from build123d import *

# Parameters (mm, degrees)
F1_DEPTH = 12.7
F3_DEPTH = 9.525
F5_DEPTH = 9.525


# Not quite as in the source:
# - a feature names something its author has since deleted; it is built from what else it names


with BuildPart() as f1:
    # F0 (on Front) → F1 (new body)
    with BuildSketch(Plane.XZ):
        Polygon((-2.1617002284, 25.4), (-14.8617002284, 25.4), (-14.8617002284, 0), (10.5382997716, 0), (10.5382997716, 12.7), (-2.1617002284, 12.7), align=None)
        Polygon((-6.2541817694, 12.4960834256), (-2.3656168028, 8.6075184589), (-3.7889303648, 3.2956399302), (-9.1008088936, 1.8723263681), (-12.9893738602, 5.7608913348), (-11.5660602982, 11.0727698635), align=None, mode=Mode.SUBTRACT)
    extrude(amount=F1_DEPTH)

    # F2 (on face) → F3 (cut)
    with BuildSketch(Plane.XY.offset(25.4)):
        Polygon((-5.7620695714, -11.1125), (-3.0124389143, -6.35), (-5.7620695714, -1.5875), (-11.2613308854, -1.5875), (-14.0109615424, -6.35), (-11.2613308854, -11.1125), align=None)
    extrude(amount=-F3_DEPTH, mode=Mode.SUBTRACT)

    # F4 (on face) → F5 (cut)
    with BuildSketch(Plane.YZ.offset(10.5382997716)):
        Polygon((-6.35, 0.850738686), (-1.5875, 3.600369343), (-1.5875, 9.099630657), (-6.35, 11.849261314), (-11.1125, 9.099630657), (-11.1125, 3.600369343), align=None)
    extrude(amount=-F5_DEPTH, mode=Mode.SUBTRACT)


solid = f1.part
For this review, take the finished solid that the model builds, in its own axes (mm). A direction names the side the tool comes from. Coordinates: 2 decimals unless noted, no trailing zeros. Order: outer loops, then holes, each group sorted by start corner. A loop starts at its lowest first (then second) coordinate and runs counter-clockwise, first axis right, second up. Notation, with made-up numbers: (47, 46.25) - (85, 46.25) arc R36 ccw to (85, 82.25) - close; hole circle Ø7 at (30, -25.5). An arc over 180 degrees is marked (long way). Answer as CSV lines item,"result". Start each with the question number.
1) Machinability: for faces 1 (the flat face through (-4.37, -4, 20.7)), 2 (the flat face through (-8.947, -6.261, 11.774)), 3 (the flat face through (1.013, -6, 6)), 4 (the flat face through (-5, 0, 13)), which of the approach directions +Z, -Z, +X, -X, +Y, -Y give a long, thin tool a straight path to every point of the face, cutting with its end or side? Answer none if there is none.
2) Insertion check: P1, Ø4, axis at x = 4, y = -7.5, coming from the +Z side; P2, Ø6.5, axis at y = -8, z = 16.5, coming from the +X side; P3, Ø5, axis at y = -6.5, z = 4, coming from the +X side. Each pin has a flat end and moves straight along its axis. Give the tip position at first contact, or say it passes through.
3) Add section A-A (x = 2). State the section outline as (y, z) points.
4) Add section D-D (z = 5.25). State the section outline as (x, y) points.
5) Add section B-B (y = -9.75). State the section outline as (x, z) points (3 decimals).
6) Draft analysis for pull direction X (two halves, no side actions). For faces 5 (the flat face through (-11.02, -6.26, 3.79)), 6 (the flat face through (10.538, -9.1, 10.5)), 7 (the flat face through (-8, -1.588, 21)), 8 (the flat face through (5.842, -8.698, 10.494)), state which applies: +X half, -X half, draft (parallel to the pull), parting line (faces both ways), or undercut.
7) To check wall thickness, follow line 1 along Y through (x, z) = (-9, 22); line 2 along Z through (x, y) = (-0.75, -0.75); line 3 along Z through (x, y) = (-8.25, -2.5) (3 decimals). State the ranges of each line that lie inside material, in increasing order. Write a range as [from, to].
8) Add section C-C (z = 22). State the section outline as (x, y) points.
Result:
1,face 1,"+Z"
1,face 2,"+Y, -Y"
1,face 3,"+X"
1,face 4,"+Z, -Z, +X, -X, +Y"
2,P1,"z = 12.7"
2,P2,"x = -2.16"
2,P3,"x = 1.01"
3,outline,"(-12.7, 0) - (0, 0) - (0, 12.7) - (-12.7, 12.7) - close; hole (-11.11, 3.6) - (-6.35, 0.85) - (-1.59, 3.6) - (-1.59, 9.1) - (-6.35, 11.85) - (-11.11, 9.1) - close"
4,outline,"(-14.86, -12.7) - (-12.48, -12.7) - (-12.48, 0) - (-14.86, 0) - close; (-3.27, -12.7) - (10.54, -12.7) - (10.54, -11.11) - (1.01, -11.11) - (1.01, -1.59) - (10.54, -1.59) - (10.54, 0) - (-3.27, 0) - close"
5,outline,"(-14.862, 0) - (10.538, 0) - (10.538, 2.814) - (1.013, 2.814) - (1.013, 9.886) - (10.538, 9.886) - (10.538, 12.7) - (-2.162, 12.7) - (-2.162, 25.4) - (-4.975, 25.4) - (-4.975, 15.875) - (-12.048, 15.875) - (-12.048, 25.4) - (-14.862, 25.4) - close; hole (-12.989, 5.761) - (-9.101, 1.872) - (-3.789, 3.296) - (-2.366, 8.608) - (-6.254, 12.496) - (-11.566, 11.073) - close"
6,face 5,"undercut"
6,face 6,"+X half"
6,face 7,"undercut"
6,face 8,"draft"
7,line 1,"[-12.7, -11.11], [-1.59, 0]"
7,line 2,"[0, 12.7]"
7,line 3,"[0, 2.1], [11.961, 15.875]"
8,outline,"(-14.86, -12.7) - (-2.16, -12.7) - (-2.16, 0) - (-14.86, 0) - close; hole (-14.01, -6.35) - (-11.26, -11.11) - (-5.76, -11.11) - (-3.01, -6.35) - (-5.76, -1.59) - (-11.26, -1.59) - close"
